```python
from build123d import *

# Parameters (mm, degrees)
SKETCH1_R           = 7.75
SKETCH1_R_2         = 2.59
BOSS_EXTRUDE1_DEPTH = 5
SKETCH2_R           = 6.5
SKETCH2_R_2         = 3.5
CUT_EXTRUDE1_DEPTH  = 2


with BuildPart() as part:
    # Sketch1 → Boss-Extrude1 (new body)
    with BuildSketch(Plane.XY):
        Circle(SKETCH1_R)
        Circle(SKETCH1_R_2, mode=Mode.SUBTRACT)
    extrude(amount=BOSS_EXTRUDE1_DEPTH)

    # Sketch2 → Cut-Extrude1 (cut)
    with BuildSketch(Plane(origin=(0, 0, 0), x_dir=(-1, 0, 0), z_dir=(0, 0, -1))):
        Circle(SKETCH2_R)
        Circle(SKETCH2_R_2, mode=Mode.SUBTRACT)
    extrude(amount=-CUT_EXTRUDE1_DEPTH, mode=Mode.SUBTRACT)


solid = part.part
```
Geometry check sheet. Reference: the model listing, model coordinates, mm. A direction names the side the tool comes from. Round coordinates to 2 decimals unless told otherwise and drop trailing zeros. Loops run counter-clockwise (first coordinate to the right, second up) from the corner with the lowest first, then second, coordinate; pieces in that order, holes last. Notation, with made-up numbers: M 22.5,-9 L 35.5,-9 A16 ccw 35.5,14 Z; hole C 19.5,-10 d7. An arc over 180 degrees is marked long. Return JSON: item names as keys, results as strings. Group by question number.
(1) Scan lines: line 1 along Y through (x, z) = (0, 2.8); line 2 along X through (y, z) = (1.25, 0.7); line 3 along Z through (x, y) = (3.25, 1.75). Record each from-to range of solid material in increasing order. Write a range as [from, to].
(2) Set-up check for faces 5 (the face through (0, -3, 5)), 6 (the face through (-3, -3, 2)): record each of +Z, -Z, +X, -X, +Y, -Y from which the full face is reachable in a straight line by a thin tool's end or side.
(3) Go/stop test with flat-tipped pins: pin 1 (3 mm diameter, centred on x = 0, y = 0, fed in from -Z); pin 2 (3 mm diameter, centred on y = 3.5, z = 1.5, fed in from -X). Record where each tip stops, or that it passes through.
(4) Section check B-B, the plane z = 0.9. Enter the section's corners in (x, y), and give its area (3 significant figures).
(5) Section check A-A, the plane y = 0. Enter the section's corners in (x, z), and give its area (3 significant figures).
(6) Section check D-D, the plane y = 5.5. Enter the section's corners in (x, z).
(7) Mould release check, pull along Y, two halves, no side actions. Record for faces 1 (the face through (-1.009, 7.684, 2.465)), 2 (the face through (0, 3, 0)), 3 (the face through (-0.56, -2.53, 2.46)), 4 (the face through (-3.233, -1.341, 0.986)): pulls with the +Y half, pulls with the -Y half, needs draft (parallel to the pull), parting line crosses it, or undercut.
Data:
{
 "1": {"line 1": "[-7.75, -2.59], [2.59, 7.75]", "line 2": "[-7.65, -6.38], [-3.27, -2.27], [2.27, 3.27], [6.38, 7.65]", "line 3": "[2, 5]"},
 "2": {"face 5": "+Z, +X, -X, +Y, -Y", "face 6": "-Z"},
 "3": {"pin 1": "through", "pin 2": "x = -7.49"},
 "4": {"outline": "C 0,0 d15.5; C 0,0 d7; hole C 0,0 d13; hole C 0,0 d5.18", "area": "73.4 mm²"},
 "5": {"outline": "M -7.75,0 L -6.5,0 L -6.5,2 L -3.5,2 L -3.5,0 L -2.59,0 L -2.59,5 L -7.75,5 Z; M 2.59,0 L 3.5,0 L 3.5,2 L 6.5,2 L 6.5,0 L 7.75,0 L 7.75,5 L 2.59,5 Z", "area": "39.6 mm²"},
 "6": {"outline": "M -5.46,0 L -3.46,0 L -3.46,2 L 3.46,2 L 3.46,0 L 5.46,0 L 5.46,5 L -5.46,5 Z"},
 "7": {"face 1": "parting line crosses it", "face 2": "needs draft", "face 3": "undercut", "face 4": "undercut"}
}
